Part model, mm, in its own coordinate system. A direction names the side the tool comes from. Round coordinates to 2 decimals unless told otherwise and drop trailing zeros. Loops run counter-clockwise (first coordinate to the right, second up) from the corner with the lowest first, then second, coordinate; pieces in that order, holes last. Notation, with made-up numbers: M 43,77.5 L 70,77.5 A21 ccw 70,115.5 Z; hole C -4.75,29 d2. An arc over 180 degrees is marked long. Put each result on its own line as item: value. Start each with the question number.
1) Slice it at D-D on x = 0. Give the cut face in (y, z).
2) Probe line 1 along Z through (x, y) = (9.35, 0); line 2 along Y through (x, z) = (9.45, 166); line 3 along Y through (x, z) = (0, 86.5). List the from-to ranges inside material, lowest first.
3) Pull direction Z, two halves, no side cores. Call faces 1 (the cylindrical face through (9.4, 0.1, 169)), 2 (the flat face through (-10, 0, 85)), 3 (the flat face through (-2, 9, 190)): +Z half, -Z half, draft (parallel to the pull), parting line (faces both ways), or undercut.
4) Slice it at B-B on z = 98.5. Give the cut face in (x, y), then the cut area to 3 significant figures.
5) Slice it at C-C on z = 166. Give the cut face in (x, y).
6) Drop flat-ended pins along their axis: pin 1 Ø1.5 at (x, y) = (0, -4) entering from +Z; pin 2 Ø8 at (y, z) = (0, 166) entering from +X. Give the stop position or say it passes through.
7) Slice it at A-A on y = 0. Give the cut face in (x, z), then the cut area to 3 significant figures.
8) Which spindle directions (+Z, -Z, +X, -X, +Y, -Y) get a long thin tool onto all of the face, cutting with end or side? Do faces 4 (the flat face through (0, 0, 0)), 5 (the flat face through (0, 10, 85)). Say none if no direction does.
```python
from build123d import *

# Parameters (mm, degrees)
SKETCH_1_W          = 20
SKETCH_1_H          = 20
SKETCH_1_R          = 9
EXTRUDE_1_DEPTH     = 190
SKETCH_2_W          = 20
SKETCH_2_H          = 20
EXTRUDE_2_DEPTH     = 22
SKETCH_4_R          = 3
CUT_EXTRUDE_2_DEPTH = 10


with BuildPart() as part:
    # 草图1 → 凸台-拉伸1 (new body)
    with BuildSketch(Plane.XY):
        Rectangle(SKETCH_1_W, SKETCH_1_H)
        Circle(SKETCH_1_R, mode=Mode.SUBTRACT)
    extrude(amount=EXTRUDE_1_DEPTH)

    # 草图2 → 凸台-拉伸2 (add)
    with BuildSketch(Plane(origin=(0, 0, 0), x_dir=(-1, 0, 0), z_dir=(0, 0, -1))):
        Rectangle(SKETCH_2_W, SKETCH_2_H)
    extrude(amount=EXTRUDE_2_DEPTH)

    # 草图4 → 切除-拉伸2 (cut)
    with BuildSketch(Plane(origin=(10, 0, 0), x_dir=(0, 0, -1), z_dir=(1, 0, 0))):
        with Locations((-166, 0)):
            Circle(SKETCH_4_R)
    extrude(amount=-CUT_EXTRUDE_2_DEPTH, mode=Mode.SUBTRACT)


solid = part.part
```
Recorded:
1. outline: M -10,-22 L 10,-22 L 10,190 L 9,190 L 9,0 L -9,0 L -9,190 L -10,190 Z
2. line 1: z = -22 to 163, 169 to 190
2. line 2: y = -10 to -3, 3 to 10
2. line 3: y = -10 to -9, 9 to 10
3. face 1: undercut
3. face 2: draft
3. face 3: +Z half
4. outline: M -10,-10 L 10,-10 L 10,10 L -10,10 Z; hole C 0,0 d18
4. area: 146 mm2
5. outline: M -10,-10 L 10,-10 L 10,-3 L 8.49,-3 A9 cw long 8.49,3 L 10,3 L 10,10 L -10,10 Z
6. pin 1: stops at z = 0
6. pin 2: stops at x = 10
7. outline: M -10,-22 L 10,-22 L 10,163 L 9,163 L 9,0 L -9,0 L -9,190 L -10,190 Z; M 9,169 L 10,169 L 10,190 L 9,190 Z
7. area: 814 mm2
8. face 4: +Z
8. face 5: +Z, -Z, +X, -X, +Y
